Design review of the part built by this model. Coordinates are the model's own, in mm. A direction names the side the tool comes from. Give positions to 0.01 mm unless a question says otherwise; leave off trailing zeros. Order: outer loops, then holes, each group sorted by start corner. A loop starts at its lowest first (then second) coordinate and runs counter-clockwise, first axis right, second up. Notation, with made-up numbers: (25.5, 49) -> (45.5, 49) arc R37 ccw to (45.5, 88) -> close; hole circle Ø4 at (12, -36.75). An arc over 180 degrees is marked (long way). One line per item, written item: value.
Solid Edge part; units mm, degrees
sketch "Sketch1" plane through (0, 0, 0) normal (0, 0, 1) x (1, 0, 0)
  line L0 (-34, -26.5) -> (34, -26.5)
  line L1 (34, -26.5) -> (34, 26.5)
  line L2 (34, 26.5) -> (-34, 26.5)
  line L3 (-34, 26.5) -> (-34, -26.5)
  dimension "D1" = 34
  dimension "D2" = 34
extrude "Ajout_matière_1" add sketch "Sketch1" along normal blind 1.5
sketch "Sketch2" plane through (0, 0, 1.5) normal (0, 0, 1) x (0, 1, 0)
  line L0 (26.5, -34) -> (26.5, -31.5)
  line L1 (26.5, -31.5) -> (13.5, -31.5)
  line L2 (13.5, -31.5) -> (11.5, -34)
  line L3 (11.5, -34) -> (26.5, -34)
  line L4 (-26.5, -34) -> (-26.5, -31.5)
  line L5 (-26.5, -31.5) -> (-24, -31.5)
  line L6 (-24, -31.5) -> (-22.5, -34)
  line L7 (-22.5, -34) -> (-26.5, -34)
  dimension "D1" = 26.5
  dimension "D2" = 26.5
  dimension "D3" = 11.5
  dimension "D4" = 26.5
  dimension "D5" = 26.5
extrude "Cutout1" cut sketch "Sketch2" against normal through all
sketch "Sketch3" plane through (0, 0, 1.5) normal (0, 0, 1) x (0, 1, 0)
  circle A0 centre (-19.5, -32) radius 1.55
  circle A1 centre (-24.5, 20.5) radius 1.505
  circle A2 centre (9, -32) radius 1.55
  circle A3 centre (24.5, 19) radius 1.505
extrude "Cutout2" cut sketch "Sketch3" against normal through all
sketch "Sketch4" plane through (0, 0, 1.5) normal (0, 0, 1) x (0, 1, 0)
  line L0 (-23.5, 23) -> (-14.5, 23)
  line L1 (-14.5, 23) -> (-14.5, 36)
  line L2 (-14.5, 36) -> (-23.5, 36)
  line L3 (-23.5, 36) -> (-23.5, 23)
  dimension "D1" = 14.5
  dimension "D2" = 23.5
extrude "Ajout_matière_2" add sketch "Sketch4" along normal blind 11
sketch "Sketch5" plane through (0, 0, 1.5) normal (0, 0, 1) x (0, 1, 0)
  line L0 (6.5, 25) -> (17.5, 25)
  line L1 (17.5, 25) -> (17.5, 41)
  line L2 (17.5, 41) -> (6.5, 41)
  line L3 (6.5, 41) -> (6.5, 25)
  dimension "D1" = 6.5
  dimension "D2" = 6.5
extrude "Ajout_matière_3" add sketch "Sketch5" along normal blind 11
sketch "Sketch6" plane through (0, 0, 1.5) normal (0, 0, 1) x (0, 1, 0)
  line L0 (-26, -31) -> (-23.5, -31)
  line L1 (-23.5, -31) -> (-23.5, 7.5)
  line L2 (-23.5, 7.5) -> (-26, 7.5)
  line L3 (-26, 7.5) -> (-26, -31)
  line L4 (23.5, 17) -> (26, 17)
  line L5 (26, 17) -> (26, -31)
  line L6 (26, -31) -> (23.5, -31)
  line L7 (23.5, -31) -> (23.5, 17)
  dimension "D1" = 26
  dimension "D2" = 26
  dimension "D3" = 23.5
  dimension "D4" = 23.5
extrude "Ajout_matière_4" add sketch "Sketch6" along normal blind 9
properties material "Acier S235"
Item 1: Add section B-B on z = 5.25. Give the boundary of the cut face in (x, y), plus the area to 3 significant figures.
Returned:
outline: (-41, 6.5) -> (-25, 6.5) -> (-25, 17.5) -> (-41, 17.5) -> close; (-36, -23.5) -> (-23, -23.5) -> (-23, -14.5) -> (-36, -14.5) -> close; (-17, 23.5) -> (31, 23.5) -> (31, 26) -> (-17, 26) -> close; (-7.5, -26) -> (31, -26) -> (31, -23.5) -> (-7.5, -23.5) -> close
area: 509 mm²
Item 2: Machinability: for faces 5 (the flat face through (31.5, -25, 1)), 6 (the flat face through (-35, -19, 1.5)), 7 (the flat face through (-33, 6.5, 7)), which of the approach directions +Z, -Z, +X, -X, +Y, -Y give a long, thin tool a straight path to every point of the face, cutting with its end or side? Answer none if there is none.
Returned:
face 5: +Z, -Z, +X, -Y
face 6: -Z, -X, +Y, -Y
face 7: +Z, +X, -X
Item 3: Add section D-D on z = 11.75. Give the boundary of the cut face in (x, y), plus the area to 3 significant figures.
Returned:
outline: (-41, 6.5) -> (-25, 6.5) -> (-25, 17.5) -> (-41, 17.5) -> close; (-36, -23.5) -> (-23, -23.5) -> (-23, -14.5) -> (-36, -14.5) -> close
area: 293 mm²
Item 4: Draft analysis for pull direction X (two halves, no side actions). For faces 1 (the cylindrical face through (30.463, 8.798, 0.76)), 2 (the cylindrical face through (30.69, -18.67, 0.76)), 3 (the flat face through (-38, 12, 1.5)), 4 (the flat face through (-34, 0, 1)), state which applies: pulls with the +X half, pulls with the -X half, needs draft (parallel to the pull), parting line crosses it, or undercut.
Returned:
face 1: undercut
face 2: undercut
face 3: needs draft
face 4: pulls with the -X half
Item 5: Add section C-C on x = 14. Give the boundary of the cut face in (y, z).
Returned:
outline: (-26.5, 0) -> (26.5, 0) -> (26.5, 1.5) -> (26, 1.5) -> (26, 10.5) -> (23.5, 10.5) -> (23.5, 1.5) -> (-23.5, 1.5) -> (-23.5, 10.5) -> (-26, 10.5) -> (-26, 1.5) -> (-26.5, 1.5) -> close
Item 6: Clearance check with flat-ended pins moving along their axes: P1, Ø2, axis at x = 10, y = -25, coming from the +Z side; P2, Ø1.6, axis at y = 20.5, z = 1, coming from the +X side; P3, Ø4.5, axis at x = 4, z = 4, coming from the +Y side. State where each tip first meets the part, or that it passes through.
Returned:
P1: z = 10.5
P2: x = 31.5
P3: y = 26
Item 7: Add section A-A on y = -19.5. Give the boundary of the cut face in (x, z).
Returned:
outline: (-36, 1.5) -> (-34, 1.5) -> (-34, 0) -> (30.45, 0) -> (30.45, 1.5) -> (-23, 1.5) -> (-23, 12.5) -> (-36, 12.5) -> close; (33.55, 0) -> (34, 0) -> (34, 1.5) -> (33.55, 1.5) -> close
Item 8: To check wall thickness, follow line 1 along X through (y, z) = (24.5, 1.2) (3 decimals); line 2 along X through (y, z) = (9, 0.8); line 3 along Y through (x, z) = (25, 5.25). State the ranges of each line that lie inside material, in increasing order. Write a range as from..to.
Returned:
line 1: -34..-20.505, -17.495..31.5
line 2: -34..30.45, 33.55..34
line 3: -26..-23.5, 23.5..26
